Part print with two shaded views. Sizes in mm from the minimum x, y, z corner. Coordinates: 2 decimals unless noted, no trailing zeros. Order: outer loops, then holes, each group sorted by start corner. A loop starts at its lowest first (then second) coordinate and runs counter-clockwise, first axis right, second up.
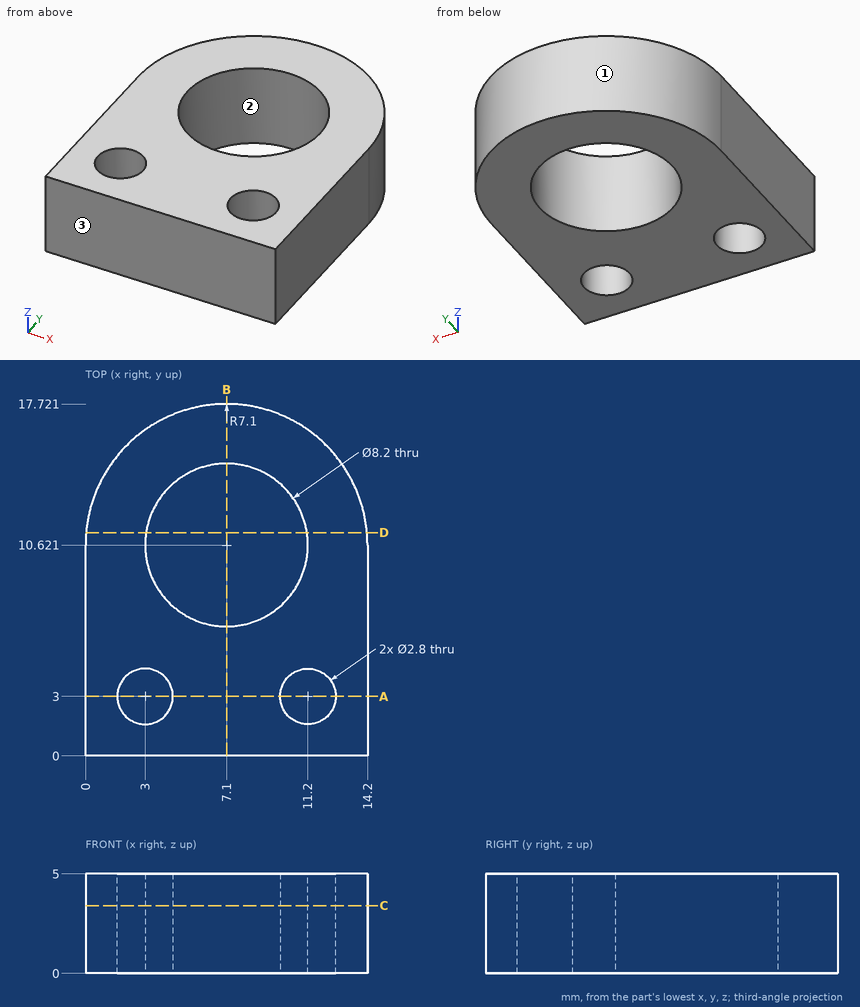
Q1. Cut at C-C on z = 3.4. Write the cut outline in (x, y).
Results list:
outline: (0, 0) - (14.2, 0) - (14.2, 10.62) arc R7.1 ccw to (0, 10.62) - close; hole circle Ø2.8 at (3, 3); hole circle Ø8.2 at (7.1, 10.62); hole circle Ø2.8 at (11.2, 3)
Q2. Pin check, flat tips, straight feed: pin 1 Ø1 at (x, z) = (4, 4) entering from +Y; pin 2 Ø3 at (x, z) = (4, 3) entering from +Y; pin 3 Ø1.7 at (x, y) = (3, 3) entering from -Z; pin 4 Ø1 at (x, z) = (12, 3) entering from +Y (1 decimal). Stop position of each tip, or through.
Results list:
pin 1: stops at y = 17.23
pin 2: stops at y = 17.54
pin 3: passes through
pin 4: stops at y = 16.2
Q3. Cut at A-A on y = 3. Write the cut outline in (x, z), and give its area (3 significant figures).
Results list:
outline: (0, 0) - (1.6, 0) - (1.6, 5) - (0, 5) - close; (4.4, 0) - (9.8, 0) - (9.8, 5) - (4.4, 5) - close; (12.6, 0) - (14.2, 0) - (14.2, 5) - (12.6, 5) - close
area: 43.0 mm2
Q4. Wall check: line 1 along Y through (x, z) = (4, 2.6) (1 decimal); line 2 along X through (y, z) = (1.75, 2.3); line 3 along X through (y, z) = (2, 1.25). Give the ranges that are in metal, low to high.
Results list:
line 1: y = 0 to 2, 4 to 7.9, 13.3 to 17
line 2: x = 0 to 2.37, 3.63 to 10.57, 11.83 to 14.2
line 3: x = 0 to 2.02, 3.98 to 10.22, 12.18 to 14.2
Q5. Cut at B-B on x = 7.1. Write the cut outline in (y, z).
Results list:
outline: (0, 0) - (6.52, 0) - (6.52, 5) - (0, 5) - close; (14.72, 0) - (17.72, 0) - (17.72, 5) - (14.72, 5) - close
Q6. Cut at D-D on y = 11.25. Write the cut outline in (x, z).
Results list:
outline: (0.03, 0) - (3.05, 0) - (3.05, 5) - (0.03, 5) - close; (11.15, 0) - (14.17, 0) - (14.17, 5) - (11.15, 5) - close
Q7. Mould opens along Y. For the marked faces 1, 2 and 3 say: pulls with the +Y half, pulls with the -Y half, needs draft (parallel to the pull), parting line crosses it, or undercut.
Results list:
face 1: pulls with the +Y half
face 2: undercut
face 3: pulls with the -Y half
